For this review, use the dimensioned drawing (mm, ordinates from the lowest corner) and the shaded views. Coordinates: 2 decimals unless noted, no trailing zeros. Write each loop counter-clockwise with the first axis right and the second up, starting at its lowest first coordinate (ties: lowest second). Pieces come first, ordered by that corner, then holes.
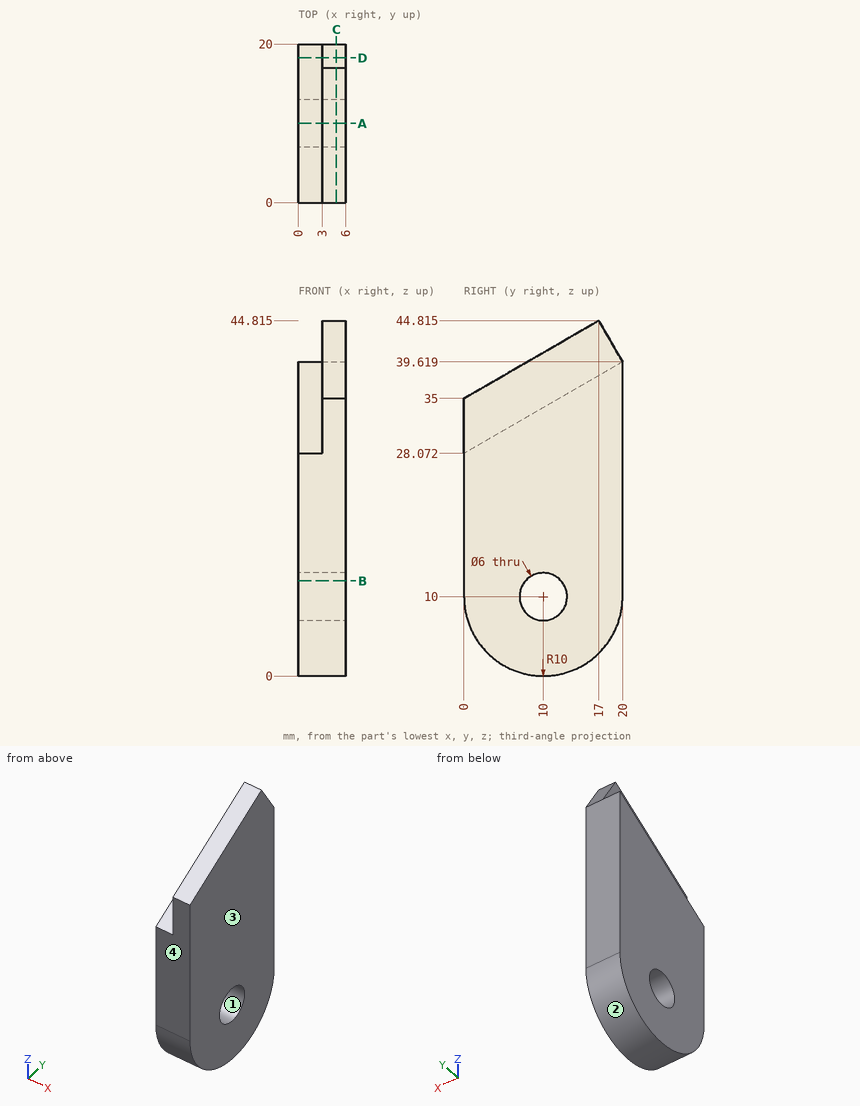
(1) Wall thickness on line 1 (Y direction, x = 3.35, z = 10); line 2 (X direction, y = 2.5, z = 34); line 3 (Z direction, x = 0.6, y = 8) (1 decimal): over which ranges is each line inside the solid? List them lowest first.
(2) Consider section A-A (y = 10). Give the boundary of the cut face in (x, z) (1 decimal), plus the area to 3 significant figures.
(3) Consider section C-C (x = 4.8). Give the boundary of the cut face in (y, z) (1 decimal), plus the area to 3 significant figures.
(4) Insertion check: pin 1 Ø2 at (x, z) = (3, 33) entering from -Y; pin 2 Ø3 at (x, y) = (1, 17.5) entering from -Z; pin 3 Ø2 at (x, y) = (3, 15.5) entering from -Z. Each pin has a flat end and moves straight along its axis. Give the tip position at first contact, or say it passes through.
(5) Consider section B-B (z = 12). Give the boundary of the cut face in (x, y).
(6) Consider section D-D (y = 18.25). Give the boundary of the cut face in (x, z), plus the area to 3 significant figures.
(7) Mouldability with a two-part tool opening along Y and no side actions: class the marked faces 1, 2, 3 and 4 as +Y half, -Y half, draft (parallel to the pull), parting line (faces both ways), or undercut.
Results:
1. line 1: y = 0 to 7, 13 to 20
1. line 2: x = 3 to 6
1. line 3: z = 0.2 to 7.8, 12.2 to 32.7
2. outline: (0, 0) - (6, 0) - (6, 7) - (0, 7) - close; (0, 13) - (6, 13) - (6, 40.8) - (3, 40.8) - (3, 33.8) - (0, 33.8) - close
2. area: 188 mm2
3. outline: (0, 10) arc R10 ccw to (20, 10) - (20, 39.6) - (17, 44.8) - (0, 35) - close; hole circle Ø6 at (10, 10)
3. area: 734 mm2
4. pin 1: stops at y = 0
4. pin 2: stops at z = 2
4. pin 3: stops at z = 1.07
5. outline: (0, 0) - (6, 0) - (6, 7.76) - (0, 7.76) - close; (0, 12.24) - (6, 12.24) - (6, 20) - (0, 20) - close
6. outline: (0, 4.35) - (6, 4.35) - (6, 42.65) - (3, 42.65) - (3, 38.61) - (0, 38.61) - close
6. area: 218 mm2
7. face 1: undercut
7. face 2: parting line
7. face 3: draft
7. face 4: -Y half
